Build history of the part. All positions in model axes, mm. A direction names the side the tool comes from. Round coordinates to 2 decimals unless told otherwise and drop trailing zeros. Loops run counter-clockwise (first coordinate to the right, second up) from the corner with the lowest first, then second, coordinate; pieces in that order, holes last. Notation, with made-up numbers: (-7, 38) - (45, 38) arc R21 cw to (45, 58) - close; hole circle Ø2 at (-13, 38). An arc over 180 degrees is marked (long way). Use a Markdown table: item, result.
Autodesk Inventor part; units mm, degrees
ref_plane "YZ Plane" through (0, 0, 0) normal (1, 0, 0) x (0, 1, 0)
ref_plane "XZ Plane" through (0, 0, 0) normal (0, 1, 0) x (-1, 0, 0)
ref_plane "XY Plane" through (0, 0, 0) normal (0, 0, 1) x (1, 0, 0)
sketch "Sketch1" plane through (0, 0, 0) normal (0, 1, 0) x (-1, 0, 0)
  line L0 (0, 0) -> (44, 0)
  line L1 (44, 0) -> (44, -300)
  line L2 (44, -300) -> (0, -300)
  line L3 (0, -300) -> (0, 0)
  dimension "d0" = 300
  dimension "d1" = 44
extrude "Extrusion1" add sketch "Sketch1" along normal blind 20
sketch "Sketch2" plane through (-44, 0, 0) normal (0, 0, 1) x (1, 0, 0)
  line L0 (44, 20) -> (0, 20)
  line L1 (44, 0) -> (0, 0)
  line L2 (0, 0) -> (44, 0)
  line L3 (44, 0) -> (44, 22)
  line L4 (44, 22) -> (0, 22)
  line L5 (0, 22) -> (0, 0)
  circle A0 centre (22, 22) radius 20.5
  dimension "d17" = 22
  dimension "d18" = 41
  dimension "d19" = 22
extrude "Extrusion2" cut sketch "Sketch2" against normal up to surface (300 mm away) contours A0 L0 | L0 A0 L4 | L4 A0
sketch "Sketch3" plane through (-44, 0, 0) normal (0, 0, 1) x (1, 0, 0)
  line L0 (0, 0) -> (0, 20)
  line L1 (0, 20) -> (44, 20)
  line L2 (44, 20) -> (44, 0)
  line L3 (44, 0) -> (0, 0)
  line L4 (0, 0) -> (0, 20)
extrude "Extrusion3" add sketch "Sketch3" against normal blind 5
sketch "Sketch4" plane through (0, 0, -300) normal (0, 0, -1) x (-1, 0, 0)
  line L0 (0, 0) -> (0, 20)
  line L1 (44, 0) -> (0, 0)
  line L2 (0, 20) -> (44, 20)
  line L3 (44, 20) -> (44, 0)
  line L4 (44, 0) -> (0, 0)
  line L5 (0, 0) -> (0, 20)
extrude "Extrusion4" add sketch "Sketch4" against normal blind 5
chamfer "Chamfer1" distance 4 angle 45 1 edges at (0, 0, -150)
chamfer "Chamfer2" distance 4 angle 45 1 edges at (-44, 0, -150)
sketch "Sketch5" plane through (0, 20, -300) normal (0, 0, -1) x (-1, 0, 0)
  line L0 (0, 0) -> (44, 0)
  line L1 (44, 0) -> (44, -20)
  line L2 (44, -20) -> (0, -20)
  line L3 (0, -20) -> (0, 0)
  line L4 (44, -16) -> (40, -20)
  line L5 (4, -20) -> (0, -16)
  line L6 (22, 0) -> (22, -20)
  line L7 (0, -10) -> (44, -10)
  line L8 (11.8539, 0) -> (11.8539, -20)
  line L9 (32.3539, 0) -> (32.3539, -20)
  line L10 (10.8539, 0) -> (10.8539, -20)
  line L11 (33.3539, 0) -> (33.3539, -20)
  line L12 (0, -9) -> (44, -9)
  circle A0 centre (11.8539, 0) radius 2
  circle A1 centre (32.3539, 0) radius 2
  point P0 (0, -20)
  point P1 (2, -18)
  point P2 (42, -18)
  point P3 (11.8539, -2)
  point P4 (10.8539, -1.7321)
  point P5 (10.8539, -10)
  point P6 (33.3539, -10)
  point P7 (33.3539, -1.7321)
  point P8 (32.3539, -2)
  point P9 (32.3539, -9)
  point P10 (11.8539, -9)
  dimension "d20" = 20
  dimension "d21" = 44
  dimension "d23" = 2
  dimension "d24" = 2
  dimension "d25" = 20.5
  dimension "d26" = 11.8539
  dimension "d27" = 1
  dimension "d28" = 1
  dimension "d29" = 9
  dimension "d30" = 4
  dimension "d31" = 4
extrude "Extrusion5" add sketch "Sketch5" along normal blind 2.5 contours A0 L8 L12 L10 | L12 L8 L7 L10 | L12 L6 L7 L8 | L12 L9 L7 L6 | A1 L11 L12 L9 | L12 L11 L7 L9
sketch "Sketch7" plane through (-33.3539, 10, -300) normal (0, -1, 0) x (1, 0, 0)
  line L0 (22.5, -2.5) -> (0, -2.5)
  line L1 (0, -2.5) -> (0, -4)
  line L2 (0, -4) -> (22.5, -4)
  line L3 (22.5, -4) -> (22.5, -2.5)
  line L4 (0, 0) -> (0, -2.5)
  line L5 (22.5, -4) -> (21.5, -4)
  line L6 (21.5, -2.5) -> (22.5, -2.5)
  line L7 (22.5, -2.5) -> (22.5, -4)
  line L8 (21.5, 0) -> (21.5, -2.5)
  line L9 (3, -2.5) -> (0, -2.5)
  line L10 (0, -2.5) -> (0, -4)
  line L11 (0, -4) -> (3, -4)
  line L12 (3, -4) -> (3, -2.5)
  line L13 (22.5, -2.5) -> (0, -2.5)
  line L14 (22.5, -4) -> (19.5, -4)
  line L15 (19.5, -4) -> (19.5, -2.5)
  line L16 (19.5, -2.5) -> (22.5, -2.5)
  line L17 (22.5, -2.5) -> (22.5, -4)
  point P0 (33.3539, 300)
  point P1 (22.5, -3.25)
  point P2 (19.5, -4)
  point P3 (19.5, -2.5)
  point P4 (3, -4)
  dimension "d36" = 1.5
  dimension "d37" = 3
  dimension "d38" = 3
extrude "Extrusion6" add sketch "Sketch7" against normal blind 3 contours L15 L2 L12 L0
extrude "Extrusion7" add sketch "Sketch7" against normal blind 9 contours L3 L2 L15 L0 | L12 L2 L1 L0
sketch "Sketch8" plane through (0, 0, 0) normal (0, -1, 0) x (1, 0, 0)
  line L0 (-44, -300) -> (-40, -300)
  line L1 (-40, -300) -> (-35, -300)
  line L2 (-35, -300) -> (-35, -290)
  line L3 (-35, -290) -> (-40, -290)
  line L4 (-40, -290) -> (-40, -300)
  line L5 (-4, 0) -> (-4, -300)
  point P0 (0, 0)
  point P1 (-37.5, -290)
  dimension "d43" = 10
  dimension "d44" = 5
extrude "Extrusion8" add sketch "Sketch8" along normal blind 6
sketch "Sketch9" plane through (-40, -6, -300) normal (-1, 0, 0) x (0, 0, 1)
  point P0 (300, 6)
  point P1 (5.0353, 2.5819)
hole "Hole1" at (-40, -3.4181, -294.9647) direction (1, 0, 0) diameter 3.5 end through all
sketch "Sketch10" plane through (-40, -6, -300) normal (-1, 0, 0) x (0, 0, 1)
  line L0 (10, 6) -> (0, 6)
  line L1 (0, 0) -> (10, 0)
  arc A0 (10, 6) -> (7.7341, 0) centre (16.1486, 0.2502) ccw
  arc A1 (5, 0) -> (8.2733, 3.2242) centre (4.0632, 4.2247) ccw
  line L2 (0, 6) -> (0, 0)
  arc A2 (2.2659, 0) -> (0, 6) centre (-6.1486, 0.2502) ccw
  arc A3 (1.7267, 3.2242) -> (5, 0) centre (5.9368, 4.2247) ccw
  line L3 (10, 6) -> (10, 0)
  point P0 (300, 6)
  point P1 (1.7267, 3.2242)
  point P2 (8.0453, 2.531)
  dimension "d54" = 8.4182
  dimension "d55" = 8.4182
  dimension "d56" = 4.3273
  dimension "d57" = 4.3273
  dimension "d58" = 2.2659
  dimension "d59" = 2.2659
  dimension "d60" = 5.9368
  dimension "d61" = 3.2242
  dimension "d64" = 1.7267
extrude "Extrusion10" cut sketch "Sketch10" against normal blind 6 contours L3 L1 A0 A1 | A2 A3 L1 L2 | A0 L1 A1 | A2 A3 L1
fillet "Fillet1" radius 2 1 edges at (-37.5, -6, -295)
sketch "Sketch11" plane through (0, 0, 0) normal (0, -1, 0) x (1, 0, 0)
  line L0 (-40, -290) -> (-40, 0)
  line L1 (-4, 0) -> (-4, -300)
  line L2 (-40, -175) -> (-4, -175)
  line L3 (-4, -175) -> (-4, -125)
  line L4 (-4, -125) -> (-40, -125)
  line L5 (-40, -125) -> (-40, -175)
  line L6 (-40, 0) -> (-4, 0)
  line L7 (-4, -300) -> (-35, -300)
  point P0 (0, 0)
  point P1 (-4, -175)
  dimension "d68" = 125
  dimension "d69" = 125
extrude "Extrusion11" add sketch "Sketch11" along normal blind 25 contours L0 L4 L1 L2
sketch "Sketch12" plane through (-40, -25, -175) normal (-1, 0, 0) x (0, 0, 1)
  point P0 (175, 25)
sketch "Sketch13" plane through (-40, -25, -175) normal (-1, 0, 0) x (0, 0, 1)
  line L0 (0, 25) -> (50, 25)
  line L1 (15, 25) -> (15, -0.9364)
  line L2 (35, 25) -> (35, -1.0252)
  line L3 (0, 25) -> (0, 0)
  line L4 (50, 25) -> (50, 0)
  arc A0 (50, 25) -> (35, -1.0252) centre (65, -0.9808) ccw
  line L5 (50, 0) -> (0, 0)
  arc A1 (25, 0) -> (39.0081, 14) centre (12.736, 26.2792) ccw
  line L6 (25, 25) -> (25, 0)
  arc A2 (15, -0.9364) -> (0, 25) centre (-15, -0.9808) ccw
  arc A3 (10.9919, 14) -> (25, 0) centre (37.264, 26.2792) ccw
  circle A4 centre (25, 12.5) radius 11.1
  arc A5 (16.7638, 5.7671) -> (33.2362, 5.7671) centre (25, 12.5) ccw
  arc A6 (12.1596, 11.7613) -> (37.8404, 11.7613) centre (25, 12.89) ccw
  point P0 (175, 25)
  point P1 (35, 0)
  point P2 (35.016, 0)
  point P3 (12.1596, 11.7613)
  point P4 (15, 7.6965)
  point P5 (19.2677, 3.5386)
  point P6 (30.7323, 3.5386)
  point P7 (35, 7.6965)
  point P8 (15, 0)
  point P9 (14.984, 0)
  point P10 (35, -0.9364)
  point P11 (25, 0)
  point P12 (14.2174, 5.8269)
  point P13 (35, 7.6823)
  point P14 (15, 7.6823)
  dimension "d73" = 15
  dimension "d74" = 15
  dimension "d75" = 29
  dimension "d76" = 30
  dimension "d77" = 14
  dimension "d78" = 22.2
extrude "Extrusion12" cut sketch "Sketch13" against normal through all contours A2 A3 A6 L5 L3 | A2 A3 | A4 L6 A5 A3 L1 | L1 A3 A4 | A2 A6 L1 L5 | A4 L2 A1 A5 L6 | A3 A5 A4 L1 | L1 A4 A3 | L1 A6 L5 | L4 L5 A0 A6 A1 | A4 A1 L2 | A5 A1 A4 L6 | L6 A4 A3 A5 | A3 A5 | A6 L2 L5 | A1 A0 | A1 A4 L2 | L2 A4 A1 A5 | A1 A5 | L5 A0 L2 | L2 A6 A0 L5
sketch "Sketch14" plane through (0, 20, -300) normal (0, 0, -1) x (-1, 0, 0)
  line L0 (1.5978, 0) -> (42.4022, 0)
  line L1 (18, 0) -> (26, 0)
  line L2 (26, 0) -> (26, -2)
  line L3 (26, -2) -> (18, -2)
  line L4 (18, -2) -> (18, 0)
  line L5 (0, -16) -> (0, 0)
  line L6 (44, -16) -> (44, 0)
  point P0 (0, -20)
  point P1 (18, -1)
  point P2 (26, 0)
  dimension "d81" = 18
  dimension "d82" = 18
  dimension "d83" = 2
extrude "Extrusion13" cut sketch "Sketch14" against normal blind 10
ref_plane "Work Plane1" through (7.9584, 20, -110) normal (0, 0, 1) x (-1, 0, 0)
split_face "Split3"
properties part number "profilrampa"
Q1. Probe line 1 (Y direction, x = -23, z = -150); line 2 (Z direction, x = -7.5, y = 13); line 3 (Y direction, x = -16.5, z = -150). List the from-to ranges inside material, lowest first.
Results found:
| item | result |
|---|---|
| line 1 | y = -25 to -23.6, -1.4 to 1.52 |
| line 2 | z = -300 to -295, -5 to 0 |
| line 3 | y = -25 to -23.6, -1.4 to 2.25 |
Q2. Cut at B-B, the plane y = -9. List the corners of the cut face in (x, z), plus the area to 3 significant figures.
Results found:
| item | result |
|---|---|
| outline | (-40, -165.27) - (-4, -165.27) - (-4, -160.53) - (-40, -160.53) - close; (-40, -139.47) - (-4, -139.47) - (-4, -134.73) - (-40, -134.73) - close |
| area | 341 mm2 |
Q3. Cut at C-C, the plane z = -195.5. List the corners of the cut face in (x, y), plus the area to 3 significant figures.
Results found:
| item | result |
|---|---|
| outline | (-44, 4) - (-40, 0) - (-4, 0) - (0, 4) - (0, 20) - (-1.6, 20) arc R20.5 cw to (-42.4, 20) - (-44, 20) - close |
| area | 286 mm2 |
Q4. Drop flat-ended pins along their axis: pin 1 (10 mm diameter, centred on x = -29.5, y = -15.5, fed in from -Z); pin 2 (4.5 mm diameter, centred on y = 15.5, z = -302.5, fed in from -X); pin 3 (2.5 mm diameter, centred on x = -23.5, y = 15, fed in from +Z); pin 4 (12.5 mm diameter, centred on y = -11.5, z = -161.5, fed in from +X). Give the stop position or say it passes through.
Results found:
| item | result |
|---|---|
| pin 1 | stops at z = -164.3 |
| pin 2 | stops at x = -33.35 |
| pin 3 | stops at z = 0 |
| pin 4 | stops at x = -4 |
Q5. Pull direction X, two halves, no side cores. Call faces 1 (the face through (-22, 8, -300)), 2 (the face through (-22, 0, -237)), 3 (the face through (-35, -1, -295)): pulls with the +X half, pulls with the -X half, needs draft (parallel to the pull), parting line crosses it, or undercut.
Results found:
| item | result |
|---|---|
| face 1 | undercut |
| face 2 | needs draft |
| face 3 | pulls with the +X half |
Q6. Cut at A-A, the plane z = -150. List the corners of the cut face in (x, y).
Results found:
| item | result |
|---|---|
| outline | (-44, 4) - (-40, 0) - (-40, -1.4) - (-4, -1.4) - (-4, 0) - (0, 4) - (0, 20) - (-1.6, 20) arc R20.5 cw to (-42.4, 20) - (-44, 20) - close; (-40, -25) - (-4, -25) - (-4, -23.6) - (-40, -23.6) - close |
Q7. Cut at D-D, the plane y = -20.5. List the corners of the cut face in (x, z).
Results found:
| item | result |
|---|---|
| outline | (-40, -159.79) - (-4, -159.79) - (-4, -157.69) - (-40, -157.69) - close; (-40, -142.31) - (-4, -142.31) - (-4, -140.21) - (-40, -140.21) - close |
Q8. Which spindle directions (+Z, -Z, +X, -X, +Y, -Y) get a long thin tool onto all of the face, cutting with end or side? Do faces 4 (the face through (-40, -1, -295)), 5 (the face through (-22, 0, -62)), 6 (the face through (-22, 13, -295)), 7 (the face through (-22, 18, -298)), 8 (the face through (-22, -25, -150)). Say none if no direction does.
Results found:
| item | result |
|---|---|
| face 4 | +Z, -Z, -X, -Y |
| face 5 | +Z, +X, -X, -Y |
| face 6 | +Y |
| face 7 | -Z, +Y |
| face 8 | +X, -X, -Y |
